from build123d import *

# Parameters (mm, degrees)
CUT_EXTRUDE2_START = -6.35
SKETCH3_R          = 9.525
CUT_EXTRUDE2_DEPTH = 6.35


with BuildPart() as part:
    # Sketch1 → Revolve1 (revolve)
    with BuildSketch(Plane.XY, mode=Mode.PRIVATE) as revolve1_sk:
        with BuildLine():
            Line((0.21036812, 2.059695488), (3.51305494, 2.944647755))
            Line((3.51305494, 2.944647755), (3.51305494, 9.525))
            Line((3.51305494, 9.525), (-9.18694506, 9.525))
            Line((-9.18694506, 9.525), (-25.4, 9.525))
            Line((-25.4, 9.525), (-25.4, 5.747363917))
            Line((-25.4, 5.747363917), (-6.293014916, 5.747363917))
            ThreePointArc((-6.293014916, 5.747363917), (-5.077995018, 5.505681433), (-4.047950886, 4.817427948))
            Line((-4.047950886, 4.817427948), (-2.155261469, 2.924738531))
            ThreePointArc((-2.155261469, 2.924738531), (-1.166419102, 2.264015185), (0, 2.032))
            ThreePointArc((0, 2.032), (0.106091689, 2.038953617), (0.21036812, 2.059695488))
        make_face()
    revolve(revolve1_sk.sketch.rotate(Axis((0, 0, 0), (1, 0, 0)), 90), axis=Axis((0, 0, 0), (1, 0, 0)))

    # Sketch3 → Cut-Extrude2 (cut)
    with BuildSketch(Plane(origin=(3.51305494, 0, 0), x_dir=(0, 0, -1), z_dir=(1, 0, 0)).offset(CUT_EXTRUDE2_START)):
        with Locations(Location((0, 0, 0), (0, 0, 180))):
            Circle(SKETCH3_R)
        Polygon((-5.829170486, -4.447932641), (0.937437419, -7.272176044), (6.766607905, -2.824243403), (5.829170486, 4.447932641), (-0.937437419, 7.272176044), (-6.766607905, 2.824243403), align=None, mode=Mode.SUBTRACT)
    extrude(amount=CUT_EXTRUDE2_DEPTH, mode=Mode.SUBTRACT)


solid = part.part
The model under review builds one solid part; all positions refer to its coordinate system, in mm. A direction names the side the tool comes from. Round coordinates to 2 decimals unless told otherwise and drop trailing zeros. Loops run counter-clockwise (first coordinate to the right, second up) from the corner with the lowest first, then second, coordinate; pieces in that order, holes last. Notation, with made-up numbers: M -27.5,3.25 L -12.5,3.25 A20 cw -12.5,8.25 Z; hole C 85,32.5 d2. An arc over 180 degrees is marked long. Answer as CSV lines item,"result".
1. We need section A-A (x = -7.5). Give the boundary of the cut face in (y, z) (3 decimals), plus the area to 3 significant figures.
Outcome:
outline,"C 0,0 d19.05; hole C 0,0 d11.495"
area,"181 mm2"
2. Draft analysis for pull direction Y (two halves, no side actions). For faces 1 (the face through (-2.837, 6.2, -2.3)), 2 (the face through (0.29, 5.08, 3.81)), 3 (the face through (1.15, 1.41, -1.83)), 4 (the face through (-15.71, 3.5, -4.56)), state which applies: pulls with the +Y half, pulls with the -Y half, needs draft (parallel to the pull), parting line crosses it, or undercut.
Outcome:
face 1,"needs draft"
face 2,"pulls with the +Y half"
face 3,"undercut"
face 4,"undercut"
3. We need section B-B (z = -7.25). Give the boundary of the cut face in (x, y), plus the area to 3 significant figures.
Outcome:
outline,"M -25.4,-6.18 L -2.84,-6.18 L -2.84,6.18 L -25.4,6.18 Z"
area,"279 mm2"
4. Insertion check: pin 1 Ø4 at (x, y) = (-19, -7) entering from -Z; pin 2 Ø8 at (x, y) = (-5, 6.5) entering from +Z; pin 3 Ø6 at (x, y) = (-10, 6.5) entering from -Z. Each pin has a flat end and moves straight along its axis. Give the tip position at first contact, or say it passes through.
Outcome:
pin 1,"stops at z = -8.11"
pin 2,"stops at z = 9.19"
pin 3,"stops at z = -8.86"
5. To check wall thickness, follow L1, parallel to Y at x = -15.5, z = 0 (3 decimals); L2, parallel to X at y = 4.25, z = -6; L3, parallel to Z at x = -5, y = -2.25. State the ranges of each line that lie inside material, in increasing order. Write a range as [from, to].
Outcome:
L1,"y = [-9.525, -5.747], [5.747, 9.525]"
L2,"x = [-25.4, -2.84]"
L3,"z = [-9.26, -4.99], [4.99, 9.26]"
6. We need section C-C (y = -8). Give the boundary of the cut face in (x, z), plus the area to 3 significant figures.
Outcome:
outline,"M -25.4,-5.17 L -2.84,-5.17 L -2.84,5.17 L -25.4,5.17 Z"
area,"233 mm2"
7. For faces 5 (the face through (-14.28, 9.3, -2.06)), 6 (the face through (0.3, 0.8, -6.3)), 7 (the face through (0.29, -5.08, -3.81)), 8 (the face through (0.3, -0.8, 6.3)), list the 3-axis set-ups (+Z, -Z, +X, -X, +Y, -Y) from which the entire face can be reached by the end or side of a thin tool; tool diameter is ignored.
Outcome:
face 5,"+X, -X"
face 6,"-Z, +X, +Y"
face 7,"-Z, +X, -Y"
face 8,"+Z, +X, -Y"
